```python
from build123d import *

# Parameters (mm, degrees)
SKETCH_W     = 8
SKETCH_H     = 8
PAD_DEPTH    = 14
SKETCH001_W  = 1
SKETCH001_H  = 1
PAD001_DEPTH = 0.5
SKETCH002_W  = 2
SKETCH002_H  = 1
PAD002_DEPTH = 0.5


with BuildPart() as part:
    # Sketch → Pad (new body)
    with BuildSketch(Plane.XY):
        with Locations((4, 4)):
            Rectangle(SKETCH_W, SKETCH_H)
    extrude(amount=PAD_DEPTH)

    # Sketch001 (on Face1 of Pad) → Pad001 (join)
    with BuildSketch(Plane.XZ):
        with Locations((2.5, 9.5)):
            Rectangle(SKETCH001_W, SKETCH001_H)
        with Locations((5.5, 9.5)):
            Rectangle(SKETCH001_W, SKETCH001_H)
        with Locations((2.5, 6.5)):
            Rectangle(SKETCH001_W, SKETCH001_H)
        with Locations((5.5, 6.5)):
            Rectangle(SKETCH001_W, SKETCH001_H)
    extrude(amount=PAD001_DEPTH)

    # Sketch002 (on Face1 of Pad001) → Pad002 (join)
    with BuildSketch(Plane.XZ):
        with Locations((4, 5.5)):
            Rectangle(SKETCH002_W, SKETCH002_H)
    extrude(amount=PAD002_DEPTH)


solid = part.part
```
Model file for the job. Use its own axes, mm. Round coordinates to 2 decimals unless told otherwise and drop trailing zeros. Order: outer loops, then holes, each group sorted by start corner. A loop starts at its lowest first (then second) coordinate and runs counter-clockwise, first axis right, second up. Notation, with made-up numbers: M -26.5,-14 L -6.5,-14 A4 ccw -6.5,-8 Z; hole C 23.25,81 d4. An arc over 180 degrees is marked long. Use CSV: the item, a comma, the result in double quotes.
Item 1: Pin check, flat tips, straight feed: pin 1 (0.6 mm diameter, centred on y = -0.5, z = 9.5, fed in from -X); pin 2 (0.6 mm diameter, centred on y = -0.5, z = 6.5, fed in from +X); pin 3 (0.6 mm diameter, centred on x = 5.5, y = -0.5, fed in from -Z). Stop position of each tip, or through.
Worked answers:
pin 1,"x = 2"
pin 2,"x = 6"
pin 3,"z = 6"
Item 2: Saw through at B-B (z = 4.5). List the corners of the cut face in (x, y), plus the area to 3 significant figures.
Worked answers:
outline,"M 0,0 L 8,0 L 8,8 L 0,8 Z"
area,"64.0 mm²"
Item 3: Probe probe 1 along Y at (x, z) = (4.25, 9). List the from-to ranges inside material, lowest first.
Worked answers:
probe 1,"0 to 8"
Item 4: Saw through at C-C (x = 1.25). List the corners of the cut face in (y, z).
Worked answers:
outline,"M 0,0 L 8,0 L 8,14 L 0,14 Z"
Item 5: Saw through at A-A (x = 5.25). List the corners of the cut face in (y, z), plus the area to 3 significant figures.
Worked answers:
outline,"M -0.5,6 L 0,6 L 0,0 L 8,0 L 8,14 L 0,14 L 0,10 L -0.5,10 L -0.5,9 L 0,9 L 0,7 L -0.5,7 Z"
area,"113 mm²"
